```python
from build123d import *

# Parameters (mm, degrees)
SKETCH1_R          = 1.6
EXTRUDE1_DEPTH     = 3
SKETCH2_R          = 1.6
CUT_EXTRUDE1_DEPTH = 10


with BuildPart() as part:
    # Sketch1 → Extrude1 (new body)
    with BuildSketch(Plane.XY):
        with BuildLine():
            Line((-45.524801784, 28.664626531), (-37.328649362, 30.860778953))
            Line((-37.328649362, 30.860778953), (-25.128844255, 23.817218191))
            ThreePointArc((-25.128844255, 23.817218191), (-23.695769789, 23.596720278), (-22.490310791, 24.402443777))
            ThreePointArc((-22.490310791, 24.402443777), (-12.321299382, 32.147149867), (0.454378412, 32.561060923))
            Line((0.454378412, 32.561060923), (0.454378412, 24.024885934))
            Line((0.454378412, 24.024885934), (-4.848291471, 19.347098838))
            ThreePointArc((-4.848291471, 19.347098838), (-8.594498853, 18.529402179), (-11.347887248, 15.860778953))
            Line((-11.347887248, 15.860778953), (-14.347887248, 10.664626531))
            Line((-14.347887248, 10.664626531), (-22.544039671, 8.468474108))
            Line((-22.544039671, 8.468474108), (-32.494200847, -8.765710592))
            ThreePointArc((-32.494200847, -8.765710592), (-34.686208494, -8.475053996), (-36.556835292, -9.654093507))
            ThreePointArc((-36.556835292, -9.654093507), (-45.724735719, -17.843308487), (-57.193646277, -22.26798145))
            ThreePointArc((-57.193646277, -22.26798145), (-59.080348228, -23.376243821), (-59.836827788, -25.429443375))
            ThreePointArc((-59.836827788, -25.429443375), (-61.709484996, -25.572317511), (-63.586979611, -25.61998316))
            Line((-63.586979611, -25.61998316), (-74.586979611, -25.61998316))
            Line((-74.586979611, -25.61998316), (-74.586979611, 4.38001684))
            Line((-74.586979611, 4.38001684), (-63.586979611, 4.38001684))
            ThreePointArc((-63.586979611, 4.38001684), (-60.086979611, 5.317839013), (-57.524801784, 7.88001684))
            Line((-57.524801784, 7.88001684), (-45.524801784, 28.664626531))
        make_face()
        with Locations((-7.860838428, 22.023527558)):
            Circle(SKETCH1_R, mode=Mode.SUBTRACT)
        with Locations((-15.617536335, 14.465529805)):
            Circle(SKETCH1_R, mode=Mode.SUBTRACT)
        with Locations((-44.255152698, 24.863723257)):
            Circle(SKETCH1_R, mode=Mode.SUBTRACT)
        with Locations((-49.098298448, 16.475148748)):
            Circle(SKETCH1_R, mode=Mode.SUBTRACT)
        with BuildLine():
            Line((-43.743844778, -0.076422397), (-40.268531978, -2.082895178))
            ThreePointArc((-40.268531978, -2.082895178), (-39.318822643, -3.369262792), (-39.615313635, -4.940498787))
            ThreePointArc((-39.615313635, -4.940498787), (-44.486377663, -10.44123439), (-50.583544918, -14.541223219))
            ThreePointArc((-50.583544918, -14.541223219), (-52.180202255, -14.627099929), (-53.329522835, -13.515456253))
            Line((-53.329522835, -13.515456253), (-54.858264001, -9.80510822))
            ThreePointArc((-54.858264001, -9.80510822), (-54.887106697, -8.355456589), (-53.928892503, -7.267271258))
            ThreePointArc((-53.928892503, -7.267271258), (-49.755509235, -4.421578878), (-46.382378242, -0.661647984))
            ThreePointArc((-46.382378242, -0.661647984), (-45.176919243, 0.144075516), (-43.743844778, -0.076422397))
        make_face(mode=Mode.SUBTRACT)
        with BuildLine():
            Line((-33.472242901, 5.540270878), (-28.472242901, 14.200524916))
            ThreePointArc((-28.472242901, 14.200524916), (-28.272442056, 15.718163006), (-29.204293709, 16.932575723))
            Line((-29.204293709, 16.932575723), (-32.668395324, 18.932575723))
            ThreePointArc((-32.668395324, 18.932575723), (-34.186033414, 19.132376568), (-35.400446131, 18.200524916))
            Line((-35.400446131, 18.200524916), (-40.400446131, 9.540270878))
            ThreePointArc((-40.400446131, 9.540270878), (-40.600246976, 8.022632788), (-39.668395324, 6.80822007))
            Line((-39.668395324, 6.80822007), (-36.204293709, 4.80822007))
            ThreePointArc((-36.204293709, 4.80822007), (-34.686655618, 4.608419225), (-33.472242901, 5.540270878))
        make_face(mode=Mode.SUBTRACT)
    extrude(amount=EXTRUDE1_DEPTH)

    # Sketch2 → Cut-Extrude1 (cut)
    with BuildSketch(Plane(origin=(0, 0, 0), x_dir=(-1, 0, 0), z_dir=(0, 0, -1))):
        with Locations((68.700777825, -0.059973733)):
            Circle(SKETCH2_R)
        with Locations((68.620801918, -7.591809129)):
            Circle(SKETCH2_R)
        with Locations((68.620801918, -20.85197665)):
            Circle(SKETCH2_R)
    extrude(amount=-CUT_EXTRUDE1_DEPTH, mode=Mode.SUBTRACT)


solid = part.part
```
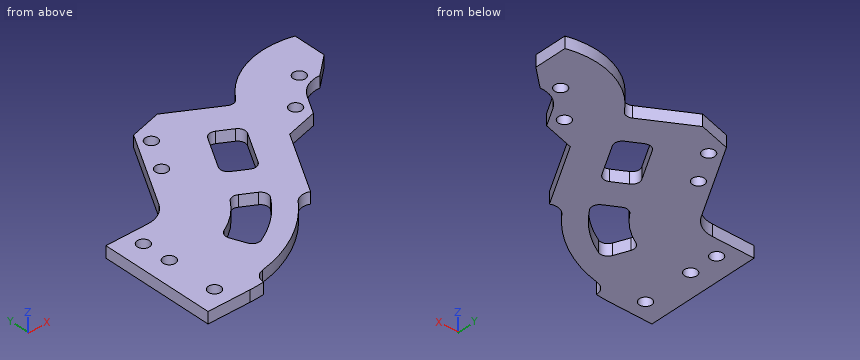
The listing builds one solid part. Answer for the finished solid, in the listing's coordinates (mm). Coordinates: 2 decimals unless noted, no trailing zeros. Loops run counter-clockwise (first coordinate to the right, second up) from the corner with the lowest first, then second, coordinate; pieces in that order, holes last. Notation, with made-up numbers: (57, 23) -> (108, 23) arc R13 cw to (108, 35) -> close; hole circle Ø4 at (9, 31.5). An arc over 180 degrees is marked (long way). Use one line per item in the form item = value. Start each with the question number.
Item 1: The part is cut by section C-C on z = 0.7. Count the separate pieces of the cut face and the enclosed holes in it, then the cut area to 3 significant figures.
Item 2: Consider L1, parallel to Y at x = -45, z = 1.8; L2, parallel to X at y = -7.5, z = 1.5; L3, parallel to Y at x = -47, z = 0.95. Determine where each line is inside the solid, lowest interval first. Write a range as [from, to].
Item 3: Flat-ended cylindrical pins translate along their axes: pin 1 Ø2.5 at (x, y) = (-68.7, -0.06) entering from -Z; pin 2 Ø1.5 at (x, z) = (-70, 2) entering from +Y; pin 3 Ø1.5 at (y, z) = (-16, 2) entering from +X; pin 4 Ø1 at (x, z) = (-44.5, 1.5) entering from -Y. Find the tip coordinate at first contact, or state that the pin passes through.
Item 4: The part is cut by section B-B on x = -30.5. Determine the outline of the cut face in (y, z), then the cut area to 3 significant figures.
Item 5: The part is cut by section A-A on y = -11.5. Determine the outline of the cut face in (x, z), then the cut area to 3 significant figures.
Answer key:
q1.separate_pieces = 1
q1.enclosed_holes = 9
q1.area = 1,850 mm2
q2.L1 = [-17.39, -10.88], [0.18, 23.45], [26.28, 28.81]
q2.L2 = [-74.59, -70.22], [-67.02, -54.28], [-41.57, -31.76]
q2.L3 = [-18.59, -12.41], [-1.5, 26.11]
q3.pin_1 = through
q3.pin_2 = 4.38
q3.pin_3 = -42.05
q3.pin_4 = -17.39
q4.outline = (-5.31, 0) -> (10.69, 0) -> (10.69, 3) -> (-5.31, 3) -> close; (17.68, 0) -> (26.92, 0) -> (26.92, 3) -> (17.68, 3) -> close
q4.area = 75.7 mm2
q5.outline = (-74.59, 0) -> (-54.16, 0) -> (-54.16, 3) -> (-74.59, 3) -> close; (-45.77, 0) -> (-38.1, 0) -> (-38.1, 3) -> (-45.77, 3) -> close
q5.area = 84.3 mm2
